Print and shaded views of the part. All mm, measured from the part's lowest x, y and z. A direction names the side the tool comes from. Round coordinates to 2 decimals unless told otherwise and drop trailing zeros. Order: outer loops, then holes, each group sorted by start corner. A loop starts at its lowest first (then second) coordinate and runs counter-clockwise, first axis right, second up. Notation, with made-up numbers: M 53.25,86.5 L 61.25,86.5 A4 cw 61.25,92.5 Z; hole C -2.75,-34.5 d2. An arc over 180 degrees is marked long. Write each question's results on one line, items separated by ' | '. Start each with the question number.
1. Which spindle directions (+Z, -Z, +X, -X, +Y, -Y) get a long thin tool onto all of the face, cutting with end or side? Do the marked faces 1, 2, 3 and 4. Say none if no direction does.
2. Band-saw the part on B-B, the plane z = 4.5. List the corners of the cut face in (x, y) (1 decimal), then the cut area to 3 significant figures.
3. Band-saw the part on D-D, the plane x = 30.5. List the corners of the cut face in (y, z) (1 decimal), then the cut area to 3 significant figures.
4. Probe L1, parallel to X at y = 13.75, z = 2.75; L2, parallel to Z at x = 15.5, y = 16.5; L3, parallel to X at y = 7.5, z = 4.75 (1 decimal). List the from-to ranges inside material, lowest first. Write a range as [from, to].
5. Band-saw the part on A-A, the plane z = 7.75. List the corners of the cut face in (x, y) (1 decimal), then the cut area to 3 significant figures.
6. Band-saw the part on C-C, the plane y = 10.5. List the corners of the cut face in (x, z) (1 decimal).
7. Drop flat-ended pins along their axis: pin 1 Ø9 at (x, y) = (3.5, 6) entering from -Z; pin 2 Ø4.5 at (y, z) = (8, 8) entering from +X; pin 3 Ø2.5 at (y, z) = (7.5, 12) entering from -X (1 decimal); pin 4 Ø3 at (y, z) = (15, 10.5) entering from -X. Give the stop position or say it passes through.
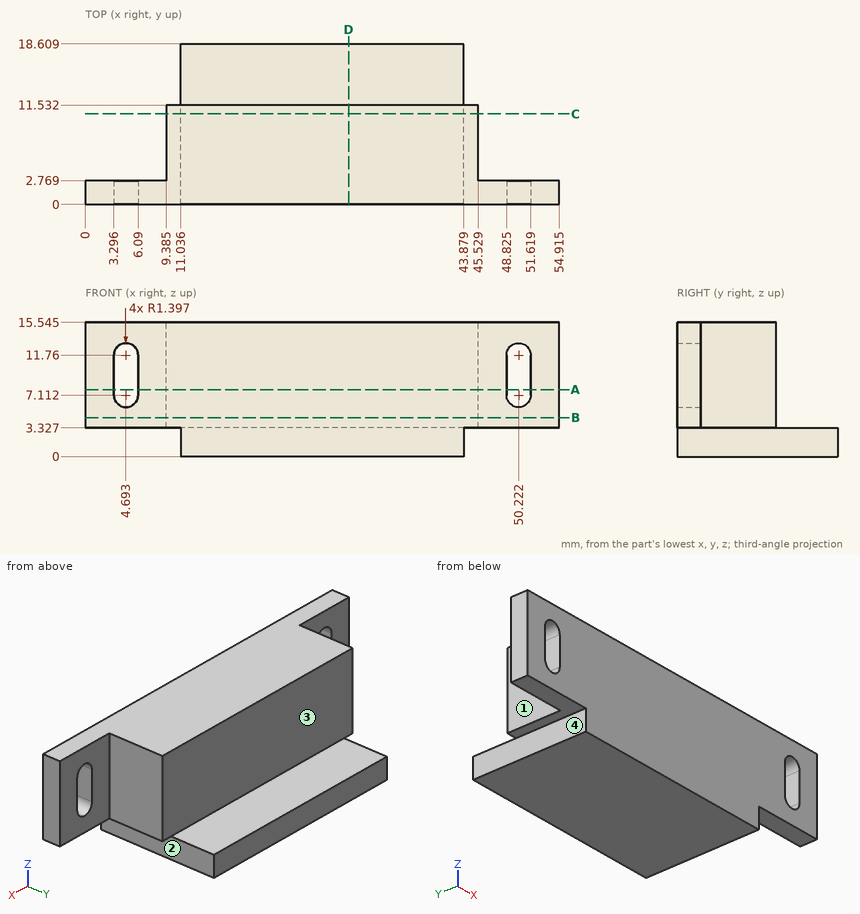
Solution:
1) face 1: +Z, -Z, -X, +Y | face 2: -Z, +X, +Y, -Y | face 3: +Z, +X, -X, +Y | face 4: -Z, -X, +Y, -Y
2) outline: M 0,0 L 54.9,0 L 54.9,2.8 L 45.5,2.8 L 45.5,11.5 L 9.4,11.5 L 9.4,2.8 L 0,2.8 Z | area: 469 mm^2
3) outline: M 0,0 L 18.6,0 L 18.6,3.3 L 11.5,3.3 L 11.5,15.5 L 0,15.5 Z | area: 203 mm^2
4) L1: [11.04, 43.88] | L2: [0, 3.33] | L3: [9.4, 45.5]
5) outline: M 0,0 L 3.3,0 L 3.3,2.8 L 0,2.8 Z; M 6.1,0 L 48.8,0 L 48.8,2.8 L 45.5,2.8 L 45.5,11.5 L 9.4,11.5 L 9.4,2.8 L 6.1,2.8 Z; M 51.6,0 L 54.9,0 L 54.9,2.8 L 51.6,2.8 Z | area: 453 mm^2
6) outline: M 9.4,3.3 L 11,3.3 L 11,0 L 43.9,0 L 43.9,3.3 L 45.5,3.3 L 45.5,15.5 L 9.4,15.5 Z
7) pin 1: z = 3.33 | pin 2: x = 45.53 | pin 3: x = 9.4 | pin 4: through
